from build123d import *

# Parameters (mm, degrees)
F0_W      = 88.9
F0_H      = 38.1
F1_DEPTH  = 53.34
F2_W      = 12.7
F2_H      = 25.4
F3_DEPTH  = 53.341
F4_W      = 25.4
F4_H      = 25.4
F5_DEPTH  = 53.341
F6_W      = 50.8
F6_H      = 12.7
F7_DEPTH  = 6.35
F9_W      = 12.7
F9_H      = 12.7
F8_W      = 12.7
F8_H      = 12.7
F10_DEPTH = 6.35
F11_R     = 6.35
F12_DEPTH = 53.341


with BuildPart() as f1:
    # F0 (on Front) → F1 (new body)
    with BuildSketch(Plane.XZ):
        Rectangle(F0_W, F0_H)
    extrude(amount=F1_DEPTH)

    # F2 (on face) → F3 (cut, through all)
    with BuildSketch(Plane.XZ.offset(53.34)):
        with Locations((-38.1, 6.35)):
            Rectangle(F2_W, F2_H)
    extrude(amount=-F3_DEPTH, mode=Mode.SUBTRACT)

    # F4 (on face) → F5 (cut, through all)
    with BuildSketch(Plane.XZ.offset(53.34)):
        with Locations((31.75, 6.35)):
            Rectangle(F4_W, F4_H)
    extrude(amount=-F5_DEPTH, mode=Mode.SUBTRACT)

    # F6 (on face) → F7 (join)
    with BuildSketch(Plane.XY.offset(19.05)):
        with Locations((-6.35, -6.35)):
            Rectangle(F6_W, F6_H)
        with Locations((-6.35, -46.99)):
            Rectangle(F6_W, F6_H)
    extrude(amount=F7_DEPTH)

    # F9 (on face) + F8 (on face) → F10 (join)
    with BuildSketch(Plane.XY.offset(25.4)):
        with Locations((-25.4, -46.99)):
            Rectangle(F9_W, F9_H)
        with Locations((12.7, -46.99)):
            Rectangle(F9_W, F9_H)
    with BuildSketch(Plane.XY.offset(25.4)):
        with Locations((-25.4, -6.35)):
            Rectangle(F8_W, F8_H)
        with Locations((12.7, -6.35)):
            Rectangle(F8_W, F8_H)
    extrude(amount=F10_DEPTH)

    # F11 (on face) → F12 (cut, through all)
    with BuildSketch(Plane.XZ.offset(53.34)):
        with Locations((-6.35, -6.35)):
            Circle(F11_R)
    extrude(amount=-F12_DEPTH, mode=Mode.SUBTRACT)


solid = f1.part
Work out the finished part from the listing and answer in its coordinate system (mm). A direction names the side the tool comes from. Coordinates: 2 decimals unless noted, no trailing zeros. Order: outer loops, then holes, each group sorted by start corner. A loop starts at its lowest first (then second) coordinate and runs counter-clockwise, first axis right, second up. Notation, with made-up numbers: (33.5, 22.25) - (51.5, 22.25) arc R19 cw to (51.5, 45.25) - close; hole circle Ø2 at (-26.75, -10). An arc over 180 degrees is marked (long way). Put each result on its own line as item: value. Start each with the question number.
1) Flat-ended cylindrical pins translate along their axes: pin 1 (4 mm diameter, centred on x = -41, y = -39, fed in from +Z); pin 2 (7 mm diameter, centred on y = -48, z = 28, fed in from -X); pin 3 (14 mm diameter, centred on x = -0.5, y = -3.5, fed in from +Z); pin 4 (7 mm diameter, centred on y = -3, z = 27.5, fed in from +X). Find the tip coordinate at first contact, or state that the pin passes through.
2) Find section B-B (y = -44). Give the vertices of the cut face in (x, z).
3) Find section A-A (x = -6.35). Give the vertices of the cut face in (y, z), plus the area to 3 significant figures.
4) For a pull along Y with two mould halves and no side action, classify faces 1 (the flat face through (-7, -40.64, 24)), 2 (the flat face through (-7, -26, 19.05)), 3 (the flat face through (-25, -6, 31.75)), 4 (the flat face through (-11, -53.34, 0)) as released by +Y, released by -Y, zero draft, split by the parting line, or undercut.
5) For faces 5 (the flat face through (-7, -12.7, 24)), 6 (the flat face through (-7, -6, 25.4)), 7 (the flat face through (19.05, -27, 8)), 8 (the flat face through (-31.75, -27, 8)), 9 (the cylindrical face through (-0.484, -27.043, -8.782)), determine the directions among +Z, -Z, +X, -X, +Y, -Y from which every point of the face is accessible in a straight line to the end or side of a thin tool.
6) Find section C-C (z = 28). Give the vertices of the cut face in (x, y).
7) Find section D-D (z = -2). Give the vertices of the cut face in (x, y), plus the area to 3 significant figures.
8) Find the intervals of material crossed by line 1 (Z direction, x = -6.35, y = -17.5); line 2 (Z direction, x = -6, y = -6.5); line 3 (Y direction, x = 4, z = 20.5), in increasing order. Write a range as from..to.
Results list:
1. pin 1: stops at z = -6.35
1. pin 2: stops at x = -31.75
1. pin 3: stops at z = 31.75
1. pin 4: stops at x = 19.05
2. outline: (-44.45, -19.05) - (44.45, -19.05) - (44.45, -6.35) - (19.05, -6.35) - (19.05, 31.75) - (6.35, 31.75) - (6.35, 25.4) - (-19.05, 25.4) - (-19.05, 31.75) - (-31.75, 31.75) - (-31.75, -6.35) - (-44.45, -6.35) - close; hole circle Ø12.7 at (-6.35, -6.35)
3. outline: (-53.34, -19.05) - (0, -19.05) - (0, -12.7) - (-53.34, -12.7) - close; (-53.34, 0) - (0, 0) - (0, 25.4) - (-12.7, 25.4) - (-12.7, 19.05) - (-40.64, 19.05) - (-40.64, 25.4) - (-53.34, 25.4) - close
3. area: 1,520 mm^2
4. face 1: undercut
4. face 2: undercut
4. face 3: zero draft
4. face 4: released by -Y
5. face 5: +Z, +X, -X
5. face 6: +Z, +Y, -Y
5. face 7: +Z, +X, +Y, -Y
5. face 8: +Z, -X, +Y, -Y
5. face 9: +Y, -Y
6. outline: (-31.75, -53.34) - (-19.05, -53.34) - (-19.05, -40.64) - (-31.75, -40.64) - close; (-31.75, -12.7) - (-19.05, -12.7) - (-19.05, 0) - (-31.75, 0) - close; (6.35, -53.34) - (19.05, -53.34) - (19.05, -40.64) - (6.35, -40.64) - close; (6.35, -12.7) - (19.05, -12.7) - (19.05, 0) - (6.35, 0) - close
7. outline: (-31.75, -53.34) - (-10.98, -53.34) - (-10.98, 0) - (-31.75, 0) - close; (-1.72, -53.34) - (19.05, -53.34) - (19.05, 0) - (-1.72, 0) - close
7. area: 2,220 mm^2
8. line 1: z = -19.05..-12.7, 0..19.05
8. line 2: z = -19.05..-12.69, -0.01..25.4
8. line 3: y = -53.34..-40.64, -12.7..0
